Could you check a few things on this model? Use its own coordinates, in mm. Face numbers are marked on the shaded views. A direction names the side the tool comes from. Give positions to 0.01 mm unless a question says otherwise; leave off trailing zeros. Write each loop counter-clockwise with the first axis right and the second up, starting at its lowest first coordinate (ties: lowest second). Pieces come first, ordered by that corner, then holes. Notation, with made-up numbers: (65.25, 35) -> (118.25, 35) arc R29 cw to (118.25, 72) -> close; hole circle Ø10 at (51.5, -25.75). An arc over 180 degrees is marked (long way). One line per question, with ' | ' between items.
from build123d import *

# Parameters (mm, degrees)
BOSS_EXTRUDE1_DEPTH = 250
SKETCH3_R           = 10
CUT_EXTRUDE1_DEPTH  = 251
SKETCH4_W           = 4
SKETCH4_H           = 4
CUT_EXTRUDE2_DEPTH  = 251
LPATTERN1_COUNT     = 10
LPATTERN1_PITCH     = 16
SKETCH5_W           = 11.978375281
SKETCH5_H           = 100
BOSS_EXTRUDE2_DEPTH = 30
SKETCH6_R           = 10
CUT_EXTRUDE3_DEPTH  = 20


with BuildPart() as part:
    # Sketch1 → Boss-Extrude1 (new body)
    with BuildSketch(Plane.XY):
        with BuildLine():
            Line((15, 0), (88, 0))
            Line((88, 0), (88, 25))
            Line((88, 25), (-88, 25))
            Line((-88, 25), (-88, 0))
            Line((-88, 0), (-15, 0))
            ThreePointArc((-15, 0), (0, -15), (15, 0))
        make_face()
    extrude(amount=BOSS_EXTRUDE1_DEPTH)

    # Sketch3 → Cut-Extrude1 (cut, through all)
    with BuildSketch(Plane.XY.offset(250)):
        Circle(SKETCH3_R)
    extrude(amount=-CUT_EXTRUDE1_DEPTH, mode=Mode.SUBTRACT)

    # Sketch4 → Cut-Extrude2 (cut, through all)
    with BuildSketch(Plane.XY.offset(250)):
        with Locations((-70, 23)):
            Rectangle(SKETCH4_W, SKETCH4_H)
    cut_extrude2 = extrude(amount=-CUT_EXTRUDE2_DEPTH, mode=Mode.SUBTRACT)

    # LPattern1: Cut-Extrude2 ×10
    with Locations(*[(i * LPATTERN1_PITCH, 0, 0) for i in range(1, LPATTERN1_COUNT)]):
        add(cut_extrude2, mode=Mode.SUBTRACT)

    # Sketch5 → Boss-Extrude2 (add)
    with BuildSketch(Plane(origin=(0, 25, 0), x_dir=(1, 0, 0), z_dir=(0, 1, 0))):
        with Locations((-82.010812359, -125)):
            Rectangle(SKETCH5_W, SKETCH5_H)
    boss_extrude2 = extrude(amount=BOSS_EXTRUDE2_DEPTH)

    # Mirror1: Boss-Extrude2 across plane
    add(boss_extrude2.mirror(Plane.ZY))

    # Sketch6 → Cut-Extrude3 (cut)
    with BuildSketch(Plane.ZY.offset(88)):
        with Locations((125, 40)):
            Circle(SKETCH6_R)
    extrude(amount=-CUT_EXTRUDE3_DEPTH, mode=Mode.SUBTRACT)


solid = part.part
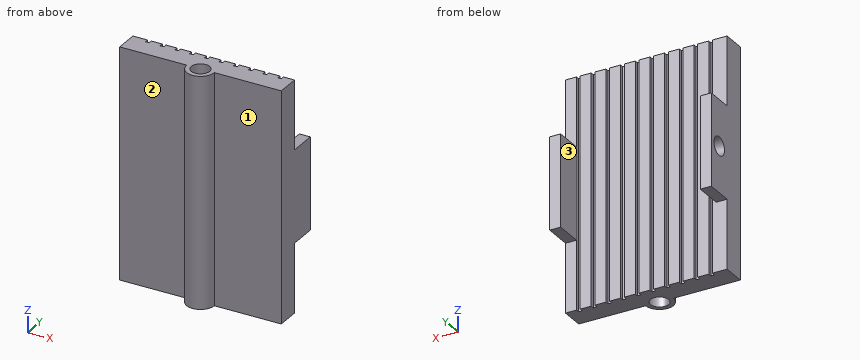
Q1. Imagine slicing it at A-A on y = 40. Please give me the cut outline in (x, z), and give its area (3 significant figures).
Answer below:
outline: (-88, 75) -> (-76.02, 75) -> (-76.02, 115) -> (-88, 115) -> close; (-88, 135) -> (-76.02, 135) -> (-76.02, 175) -> (-88, 175) -> close; (76.02, 75) -> (88, 75) -> (88, 175) -> (76.02, 175) -> close | area: 2,160 mm^2
Q2. If I drill on line 1 along Y through (x, z) = (-82, 125); line 2 along X through (y, z) = (51.5, 164.5); line 3 along Y through (x, z) = (0, 91.5), over which ranges is the centre line in solid material (lowest first)?
Answer below:
line 1: y = 0 to 30, 50 to 55 | line 2: x = -88 to -76.02, 76.02 to 88 | line 3: y = -15 to -10, 10 to 25
Q3. Will these pins go through, and if not, where does the flat tip stop? pin 1 (3 mm diameter, centred on x = 43, z = 115, fed in from -Y); pin 2 (1.5 mm diameter, centred on x = -12.5, z = 206.5, fed in from -Y); pin 3 (1.5 mm diameter, centred on x = 17.5, z = 116.5, fed in from +Y).
Answer below:
pin 1: stops at y = 0 | pin 2: stops at y = -9.32 | pin 3: stops at y = 25
Q4. Imagine slicing it at C-C on z = 125. Count the separate pieces of the cut face and the enclosed holes in it, and give its area (3 significant figures).
Answer below:
separate pieces: 2 | enclosed holes: 1 | area: 4,760 mm^2
Q5. Imagine slicing it at D-D on x = -33. Please give me the cut outline in (y, z).
Answer below:
outline: (0, 0) -> (25, 0) -> (25, 250) -> (0, 250) -> close
Q6. On a 3-axis mill with a long thin cutter (end or side, diameter ignored), from which of +Z, -Z, +X, -X, +Y, -Y can I reach the whole of each face in a straight line? I mean the marked faces 1, 2 and 3. Say none if no direction works.
Answer below:
face 1: +Z, -Z, +X, -Y | face 2: +Z, -Z, -X, -Y | face 3: +Z, -Z, +Y
Q7. Imagine slicing it at B-B on x = 0. Please give me the cut outline in (y, z).
Answer below:
outline: (-15, 0) -> (-10, 0) -> (-10, 250) -> (-15, 250) -> close; (10, 0) -> (25, 0) -> (25, 250) -> (10, 250) -> close
